Design review of the part built by this model. Coordinates are the model's own, in mm. Coordinates: 2 decimals unless noted, no trailing zeros. Write each loop counter-clockwise with the first axis right and the second up, starting at its lowest first coordinate (ties: lowest second). Pieces come first, ordered by that corner, then holes. Notation, with made-up numbers: (-39.75, -7.5) -> (11.25, -7.5) arc R21 ccw to (11.25, 19.5) -> close; hole circle Ø8 at (68.25, 49). An arc over 180 degrees is marked (long way). Return JSON: item names as keys, results as strings. Group by question number.
from build123d import *

# Parameters (mm, degrees)
SKETCH1_R           = 0.75
SKETCH1_R_2         = 7.62
BOSS_EXTRUDE1_DEPTH = 0.8


with BuildPart() as part:
    # Sketch1 → Boss-Extrude1 (new body)
    with BuildSketch(Plane.XY):
        with BuildLine():
            Line((-0.08854439, -19.128525646), (31.178350927, -19.305614409))
            ThreePointArc((31.178350927, -19.305614409), (46.900344572, -3.760709545), (31.355439708, 11.961284099))
            Line((31.355439708, 11.961284099), (0.08854439, 12.138372862))
            ThreePointArc((0.08854439, 12.138372862), (-15.633449254, -3.406532002), (-0.08854439, -19.128525646))
        make_face()
        with Locations((12.5, -3.565873621)):
            Circle(SKETCH1_R, mode=Mode.SUBTRACT)
        with Locations((0, -3.495076392)):
            Circle(SKETCH1_R_2, mode=Mode.SUBTRACT)
        with Locations((-12.5, -3.424279164)):
            Circle(SKETCH1_R, mode=Mode.SUBTRACT)
        with Locations((18.766895317, -3.601367926)):
            Circle(SKETCH1_R, mode=Mode.SUBTRACT)
        with Locations((31.266895317, -3.672165155)):
            Circle(SKETCH1_R_2, mode=Mode.SUBTRACT)
        with Locations((43.766895317, -3.742962383)):
            Circle(SKETCH1_R, mode=Mode.SUBTRACT)
        with Locations((31.196098089, -16.172165155)):
            Circle(SKETCH1_R, mode=Mode.SUBTRACT)
        with Locations((22.377999352, -12.460938719)):
            Circle(SKETCH1_R, mode=Mode.SUBTRACT)
        with Locations((40.055668882, -12.56106112)):
            Circle(SKETCH1_R, mode=Mode.SUBTRACT)
        with Locations((22.478121753, 5.21673081)):
            Circle(SKETCH1_R, mode=Mode.SUBTRACT)
        with Locations((40.155791283, 5.11660841)):
            Circle(SKETCH1_R, mode=Mode.SUBTRACT)
        with Locations((31.337692546, 8.827834845)):
            Circle(SKETCH1_R, mode=Mode.SUBTRACT)
        with Locations((8.788773564, -12.383972357)):
            Circle(SKETCH1_R, mode=Mode.SUBTRACT)
        with Locations((-0.070797229, -15.995076392)):
            Circle(SKETCH1_R, mode=Mode.SUBTRACT)
        with Locations((-8.888895965, -12.283849957)):
            Circle(SKETCH1_R, mode=Mode.SUBTRACT)
        with Locations((0.070797229, 9.004923608)):
            Circle(SKETCH1_R, mode=Mode.SUBTRACT)
        with Locations((8.888895965, 5.293697172)):
            Circle(SKETCH1_R, mode=Mode.SUBTRACT)
        with Locations((-8.788773564, 5.393819573)):
            Circle(SKETCH1_R, mode=Mode.SUBTRACT)
    extrude(amount=BOSS_EXTRUDE1_DEPTH)


solid = part.part
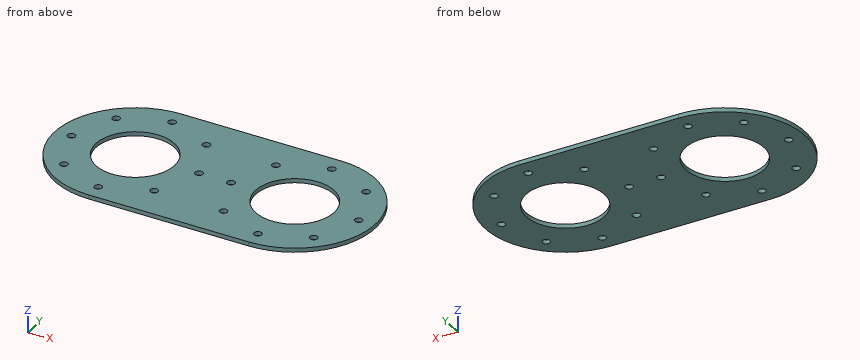
Q1. We need section C-C on z = 0.55. State how many separate pieces and enclosed holes the cut face has, plus the area to 3 significant figures.
Q2. For P1, Ø1.7, axis at x = 40.06, y = -12.56, coming from the +Z side, flat-tipped, find the tip position at first contact; note if it passes through.
Q3. We need section A-A on y = -6. Write out the cut boundary in (x, z).
Q4. Wall thickness on L1, parallel to Y at x = 0, z = 0.2; L2, parallel to X at y = -2, z = 0.3; L3, parallel to X at y = -10.5, z = 0.2: over which ranges is each line inside the solid? List them lowest first.
Q5. We need section D-D on y = 0. Write out the cut boundary in (x, z), plus the area to 3 significant figures.
Q6. We need section B-B on x = 33.5. Write out the cut boundary in (y, z), plus the area to 3 significant figures.
Findings below:
{
 "1": {"separate pieces": "1", "enclosed holes": "18", "area": "1,350 mm^2"},
 "2": {"P1": "stops at z = 0.8"},
 "3": {"outline": "(-15.43, 0) -> (-7.2, 0) -> (-7.2, 0.8) -> (-15.43, 0.8) -> close; (7.2, 0) -> (24.01, 0) -> (24.01, 0.8) -> (7.2, 0.8) -> close; (38.52, 0) -> (46.73, 0) -> (46.73, 0.8) -> (38.52, 0.8) -> close"},
 "4": {"L1": "y = -19.13 to -16.74, -15.25 to -11.12, 4.12 to 8.26, 9.75 to 12.14", "L2": "x = -15.56 to -7.47, 7.47 to 23.83, 38.7 to 46.81", "L3": "x = -13.98 to -3, 3 to 27.88, 34.65 to 45.33"},
 "5": {"outline": "(-15.24, 0) -> (-6.77, 0) -> (-6.77, 0.8) -> (-15.24, 0.8) -> close; (6.77, 0) -> (24.59, 0) -> (24.59, 0.8) -> (6.77, 0.8) -> close; (37.94, 0) -> (46.46, 0) -> (46.46, 0.8) -> (37.94, 0.8) -> close", "area": "27.8 mm^2"},
 "6": {"outline": "(-19.15, 0) -> (-10.96, 0) -> (-10.96, 0.8) -> (-19.15, 0.8) -> close; (3.61, 0) -> (11.8, 0) -> (11.8, 0.8) -> (3.61, 0.8) -> close", "area": "13.1 mm^2"}
}
